Verification items for the finished model (mm, model axes). A direction names the side the tool comes from. Round coordinates to 2 decimals unless told otherwise and drop trailing zeros. Loops run counter-clockwise (first coordinate to the right, second up) from the corner with the lowest first, then second, coordinate; pieces in that order, holes last. Notation, with made-up numbers: M 59.5,33.5 L 81.5,33.5 A11 cw 81.5,45.5 Z; hole C -36,39.5 d11. An arc over 180 degrees is marked long. One line per item, written item: value.
Autodesk Inventor part; units mm, degrees
ref_plane "YZ Plane" through (0, 0, 0) normal (1, 0, 0) x (0, 1, 0)
ref_plane "XZ Plane" through (0, 0, 0) normal (0, 1, 0) x (-1, 0, 0)
ref_plane "XY Plane" through (0, 0, 0) normal (0, 0, 1) x (1, 0, 0)
sketch "Sketch1" plane through (0, 0, 0) normal (0, 0, 1) x (1, 0, 0)
  circle A0 centre (0, 0) radius 25.4
  dimension "d0" = 50.8
extrude "Extrusion1" add sketch "Sketch1" along normal mid plane 146
sketch "Sketch2" plane through (0, 0, 0) normal (0, 1, 0) x (-1, 0, 0)
  circle A0 centre (0, 0) radius 19.05
  dimension "d3" = 38.1
extrude "Extrusion2" add sketch "Sketch2" along normal blind 66.5
shell "Shell1" thickness 1.65 removed faces 3 at (5.6226, 66.5, 0.0883) at (-7.2508, -1.9085, 73) at (-7.2508, -1.9085, -73)
properties part number "ASME BPE - RED TEE-50.8-38.1" material "Stainless Steel, 316L"
(1) Mould release check, pull along Z, two halves, no side actions. Record for faces 3 (the face through (-16.597, 40.978, -5.226)), 4 (the face through (-8.38, 66.5, -15.43)), 5 (the face through (17, -17, -73)): +Z half, -Z half, draft (parallel to the pull), parting line (faces both ways), or undercut.
Completed:
face 3: undercut
face 4: draft
face 5: -Z half
(2) Sectioned sample at D-D on x = 21.5. Enter the section's corners in (y, z), and give its area (3 significant figures).
Completed:
outline: M -13.52,-73 L -10.09,-73 L -10.09,73 L -13.52,73 Z; M 10.09,-73 L 13.52,-73 L 13.52,73 L 10.09,73 Z
area: 1,000 mm^2
(3) Thickness scan on L1, parallel to X at y = 0.5, z = 44.5; L2, parallel to Y at x = 0, z = -32; L3, parallel to X at y = 29, z = 0. Record the ranges inside material, lowest first. Write a range as from..to.
Completed:
L1: x = -25.4..-23.74, 23.74..25.4
L2: y = -25.4..-23.75, 23.75..25.4
L3: x = -19.05..-17.4, 17.4..19.05
(4) Sectioned sample at B-B on y = 0. Enter the section's corners in (x, z).
Completed:
outline: M -25.4,-73 L -23.75,-73 L -23.75,73 L -25.4,73 Z; M 23.75,-73 L 25.4,-73 L 25.4,73 L 23.75,73 Z
(5) Sectioned sample at A-A on x = 0. Enter the section's corners in (y, z).
Completed:
outline: M -25.4,-73 L -23.75,-73 L -23.75,73 L -25.4,73 Z; M 23.75,-73 L 25.4,-73 L 25.4,-19.05 L 66.5,-19.05 L 66.5,-17.4 L 23.75,-17.4 Z; M 23.75,17.4 L 66.5,17.4 L 66.5,19.05 L 25.4,19.05 L 25.4,73 L 23.75,73 Z
(6) Tool access check on faces 1 (the face through (-18.17, 41.3, -5.72)), 2 (the face through (17, -17, 73)). Record the directions out of +Z, -Z, +X, -X, +Y, -Y that give a thin tool (end or side, any length) a straight path to the whole face; none if there is none.
Completed:
face 1: +Y
face 2: +Z, +X, -X, +Y, -Y
(7) Depth check by flat-ended pin: pin 1 Ø1 at (x, z) = (17.5, 13.5) entering from -Y; pin 2 Ø8 at (y, z) = (53, -21.5) entering from -X; pin 3 Ø5 at (x, z) = (9.5, -36.5) entering from -Y. Enter the tip coordinate at first touch or a pass-through.
Completed:
pin 1: stops at y = -18.87
pin 2: stops at x = -7.53
pin 3: stops at y = -24.42
(8) Sectioned sample at C-C on z = 0. Enter the section's corners in (x, y).
Completed:
outline: M -19.05,16.8 A25.4 ccw long 19.05,16.8 L 19.05,66.5 L 17.4,66.5 L 17.4,16.16 A23.75 cw long -17.4,16.16 L -17.4,66.5 L -19.05,66.5 Z
